Work out the finished part from the listing and answer in its coordinate system (mm). Face numbers are marked on the shaded views. A direction names the side the tool comes from. Give positions to 0.01 mm unless a question says otherwise; leave off trailing zeros. Loops run counter-clockwise (first coordinate to the right, second up) from the corner with the lowest first, then second, coordinate; pieces in that order, holes last. Notation, with made-up numbers: M -31,-1 L 10,-1 A24 ccw 10,9 Z; hole C 81.5,52 d1. An arc over 180 degrees is marked long. Write item = value, one per line. Start each with the question number.
1. Consider L1, parallel to Z at x = 18.5, y = 25.5; L2, parallel to X at y = 1, z = 2; L3, parallel to Z at x = -14, y = -18.5. Determine where each line is inside the solid, lowest interval first. Write a range as [from, to].
2. For the marked faces 1, 2 and 3, determine the directions among +Z, -Z, +X, -X, +Y, -Y from which every point of the face is accessible in a straight line to the end or side of a thin tool.
3. Flat-ended cylindrical pins translate along their axes: pin 1 Ø1 at (x, z) = (10.5, 7.5) entering from -Y; pin 2 Ø4 at (x, y) = (-21, -12) entering from +Z; pin 3 Ø1.5 at (y, z) = (-13, 16) entering from -X. Find the tip coordinate at first contact, or state that the pin passes through.
4. Section D-D on z = 3.25 is taken. Determine the outline of the cut face in (x, y), plus the area to 3 significant figures.
5. Section B-B on x = -29 is taken. Determine the outline of the cut face in (y, z), plus the area to 3 significant figures.
6. Section C-C on z = 17.5 is taken. Determine the outline of the cut face in (x, y).
7. Section A-A on z = 8 is taken. Determine the outline of the cut face in (x, y), plus the area to 3 significant figures.
```python
from build123d import *

# Parameters (mm, degrees)
F0_R     = 35
F1_DEPTH = 6.35
F3_DEPTH = 12.7
F4_R     = 2.54


with BuildPart() as f1:
    # F0 (on Top) → F1 (new body)
    with BuildSketch(Plane.XY):
        Circle(F0_R)
    extrude(amount=F1_DEPTH)

    # F2 (on face) → F3 (join)
    with BuildSketch(Plane.XY.offset(6.35)):
        Polygon((18.384776, -18.384776), (26, 0), (18.384776, 18.384776), (0, 26), (-18.384776, 18.384776), (-26, 0), (-18.384776, -18.384776), (0, -26), align=None)
    extrude(amount=F3_DEPTH)

    # F4
    f4_edges = [f1.edges().sort_by_distance(p)[0] for p in [
        (22.192388, -9.192388, 19.05),
        (22.192388, 9.192388, 19.05),
        (9.192388, 22.192388, 19.05),
        (-9.192388, 22.192388, 19.05),
        (9.192388, -22.192388, 19.05),
        (-9.192388, -22.192388, 19.05),
        (-22.192388, -9.192388, 19.05),
        (-22.192388, 9.192388, 19.05),
    ]]
    fillet(f4_edges, radius=F4_R)


solid = f1.part
```
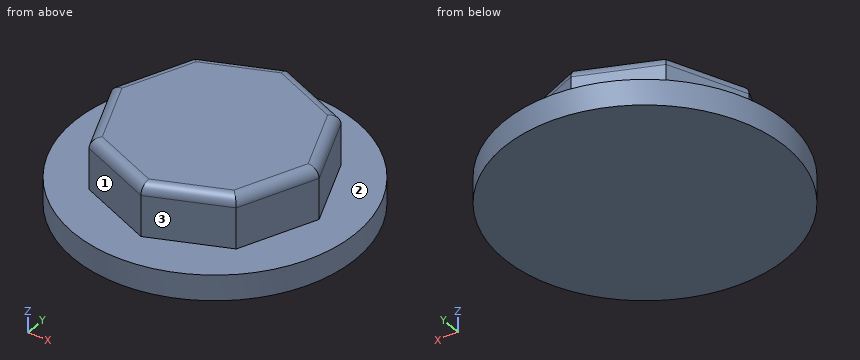
Verdict:
q1.L1 = [0, 6.35]
q1.L2 = [-34.99, 34.99]
q1.L3 = [0, 18.86]
q2.face_1 = +Z, -X, -Y
q2.face_2 = +Z
q2.face_3 = +Z, +X, -Y
q3.pin_1 = -21.86
q3.pin_2 = 19
q3.pin_3 = -20.93
q4.outline = C 0,0 d70
q4.area = 3,850 mm2
q5.outline = M -19.6,0 L 19.6,0 L 19.6,6.35 L -19.6,6.35 Z
q5.area = 249 mm2
q6.outline = M -25.78,0 L -18.23,-18.23 L 0,-25.78 L 18.23,-18.23 L 25.78,0 L 18.23,18.23 L 0,25.78 L -18.23,18.23 Z
q7.outline = M -26,0 L -18.38,-18.38 L 0,-26 L 18.38,-18.38 L 26,0 L 18.38,18.38 L 0,26 L -18.38,18.38 Z
q7.area = 1,910 mm2
